Design review of the part built by this model. Coordinates are the model's own, in mm. Coordinates: 2 decimals unless noted, no trailing zeros. Loops run counter-clockwise (first coordinate to the right, second up) from the corner with the lowest first, then second, coordinate; pieces in that order, holes last. Notation, with made-up numbers: (2, -15.5) -> (18, -15.5) arc R11 ccw to (18, 1.5) -> close; hole circle Ø5 at (49, 59). An arc over 180 degrees is marked (long way). One line per item, written item: value. Start each with the question number.
1. Add section B-B on x = -5. Write out the cut boundary in (y, z), plus the area to 3 significant figures.
2. For probe 1 along X at (y, z) = (3.5, 3.9); probe 2 along X at (y, z) = (-43, 1.9); probe 3 along Y at (x, z) = (-1.75, 1.75), list the stretches that pass through material, from the lowest coordinate up.
3. Insertion check: pin 1 (1 mm diameter, centred on x = -9.5, y = -17, fed in from -Z); pin 2 (1.5 mm diameter, centred on x = -13, z = 1.5, fed in from +Y); pin 3 (2 mm diameter, centred on y = -78, z = 2, fed in from -X); pin 4 (2.5 mm diameter, centred on y = 21, z = 1.5, fed in from -X). Each pin has a flat end and moves straight along its axis. Give the tip position at first contact, or say it passes through.
4. Add section C-C on z = 2.5. Give the number of separate pieces and of enclosed holes in the cut face, plus the area to 3 significant figures.
5. Add section A-A on y = 13. Write out the cut boundary in (x, z).
6. Add section D-D on x = -10.5. Write out the cut boundary in (y, z).
```python
from build123d import *

# Parameters (mm, degrees)
BOSS_EXTRUDE1_DEPTH = 5
FILLET1_R           = 10
FILLET2_R           = 5
SKETCH3_R           = 1.5
CUT_EXTRUDE1_DEPTH  = 15


with BuildPart() as part:
    # Sketch1 → Boss-Extrude1 (new body)
    with BuildSketch(Plane.XY):
        Polygon((4.681102362, -8.657480315), (11.681102362, -8.657480315), (11.681102362, 18.342519685), (2.681102362, 18.342519685), (2.681102362, 23.842519685), (-0.318897638, 23.842519685), (-0.318897638, 18.342519685), (-0.318897638, 15.342519685), (8.681102362, 15.342519685), (8.681102362, -5.657480315), (-12.318897638, -5.657480315), (-12.318897638, 15.342519685), (-3.318897638, 15.342519685), (-3.318897638, 18.342519685), (-3.318897638, 23.842519685), (-6.318897638, 23.842519685), (-6.318897638, 18.342519685), (-15.318897638, 18.342519685), (-15.318897638, -8.657480315), (-8.318897638, -8.657480315), (-8.318897638, -108.657480315), (4.681102362, -108.657480315), align=None)
    extrude(amount=BOSS_EXTRUDE1_DEPTH)

    # Fillet1
    # the kernel refuses this fillet: 10 mm, written as the material it adds along each edge
    with BuildSketch(Plane(origin=(-8.318897638, -8.657480315, 0), x_dir=(0, -1, 0), z_dir=(0, 0, 1))) as fillet1_piece_1:
        with BuildLine():
            CenterArc((9.539392014, -10), FILLET1_R, 90, 72.542396876)
            Line((0, -7), (-0.19078784, -6.94))
            ThreePointArc((-0.19078784, -6.94), (-0.2, -3.5), (-0.2, 0))
            Line((-0.2, 0), (0, 0.2))
            Line((0, 0.2), (9.539392014, 0.2))
            Line((9.539392014, 0.2), (9.539392014, 0))
        make_face()
    extrude(amount=5)
    with BuildSketch(Plane(origin=(4.681102362, -8.657480315, 0), x_dir=(1, 0, 0), z_dir=(0, 0, 1))) as fillet1_piece_2:
        with BuildLine():
            CenterArc((10, -9.539392014), FILLET1_R, 107.457603124, 72.542396876)
            Line((0, -9.539392014), (-0.2, -9.539392014))
            Line((-0.2, -9.539392014), (-0.2, 0))
            Line((-0.2, 0), (0, 0.2))
            ThreePointArc((0, 0.2), (3.5, 0.2), (6.94, 0.19078784))
            Line((6.94, 0.19078784), (7, 0))
        make_face()
    extrude(amount=5)

    # Fillet2
    fillet2_edges = [part.edges().sort_by_distance(p)[0] for p in [
        (4.681102362, -108.657480315, 2.5),
        (-8.318897638, -108.657480315, 2.5),
    ]]
    fillet(fillet2_edges, radius=FILLET2_R)

    # Sketch3 → Cut-Extrude1 (cut)
    with BuildSketch(Plane.ZY.offset(6.318897638)):
        with Locations(Location((2.5, 21.342519685, 0), (0, 0, 90))):
            Circle(SKETCH3_R)
    extrude(amount=-CUT_EXTRUDE1_DEPTH, mode=Mode.SUBTRACT)


solid = part.part
```
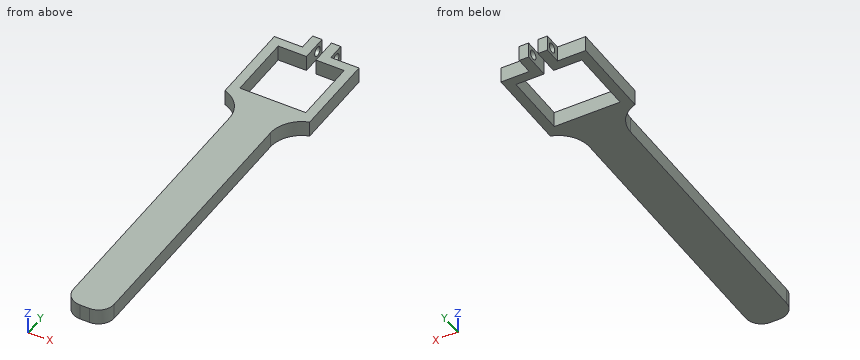
Worked answers:
1. outline: (-108.37, 0) -> (-5.66, 0) -> (-5.66, 5) -> (-108.37, 5) -> close; (15.34, 0) -> (23.84, 0) -> (23.84, 5) -> (15.34, 5) -> close; hole circle Ø3 at (21.34, 2.5)
1. area: 549 mm²
2. probe 1: x = -15.32 to -12.32, 8.68 to 11.68
2. probe 2: x = -8.32 to 4.68
2. probe 3: y = -108.66 to -5.66
3. pin 1: passes through
3. pin 2: stops at y = 18.34
3. pin 3: stops at x = -8.32
3. pin 4: stops at x = -6.32
4. separate pieces: 3
4. enclosed holes: 0
4. area: 1,620 mm²
5. outline: (-15.32, 0) -> (-12.32, 0) -> (-12.32, 5) -> (-15.32, 5) -> close; (8.68, 0) -> (11.68, 0) -> (11.68, 5) -> (8.68, 5) -> close
6. outline: (-11.96, 0) -> (-5.66, 0) -> (-5.66, 5) -> (-11.96, 5) -> close; (15.34, 0) -> (18.34, 0) -> (18.34, 5) -> (15.34, 5) -> close
